Could you check a few things on this model? Use its own coordinates, in mm. A direction names the side the tool comes from. Coordinates: 2 decimals unless noted, no trailing zeros. Loops run counter-clockwise (first coordinate to the right, second up) from the corner with the lowest first, then second, coordinate; pieces in that order, holes last.
from build123d import *

# Parameters (mm, degrees)
SKETCH_R        = 40
SKETCH_R_2      = 1.7
PAD_DEPTH       = 5
POCKET_DEPTH    = 231.496033
CHAMFER_SIZE    = 2.5
SKETCH002_W     = 4
SKETCH002_H     = 20
PAD001_DEPTH    = 24
SKETCH003_R     = 2.2
POCKET001_DEPTH = 57.501
SKETCH004_R     = 1.75
POCKET002_DEPTH = 29.001
SKETCH005_R     = 2
POCKET003_DEPTH = 4
SKETCH006_R     = 2
POCKET004_DEPTH = 4
PAD002_DEPTH    = 2.5
SKETCH008_R     = 1.75
POCKET005_DEPTH = 262.590383
SKETCH009_R     = 2.85
POCKET006_DEPTH = 3
SKETCH015_W     = 4
SKETCH015_H     = 13
PAD003_DEPTH    = 12
POCKET007_DEPTH = 4
SKETCH017_W     = 2
SKETCH017_H     = 20
PAD004_DEPTH    = 40
SKETCH018_W     = 4
SKETCH018_H     = 10
PAD005_DEPTH    = 16
SKETCH019_W     = 16
SKETCH019_H     = 4
PAD006_DEPTH    = 4
SKETCH020_W     = 8.3
SKETCH020_H     = 3.5
SKETCH020_W_2   = 7.5
SKETCH020_H_2   = 4
POCKET008_DEPTH = 2
SKETCH021_W     = 4
SKETCH021_H     = 8
POCKET009_DEPTH = 15.001


with BuildPart() as part:
    # Sketch → Pad (new body)
    with BuildSketch(Plane.XY):
        Circle(SKETCH_R)
        with Locations((10, 10)):
            Circle(SKETCH_R_2, mode=Mode.SUBTRACT)
        with Locations((-10, 10)):
            Circle(SKETCH_R_2, mode=Mode.SUBTRACT)
        with Locations((-10, -10)):
            Circle(SKETCH_R_2, mode=Mode.SUBTRACT)
        with Locations((10, -10)):
            Circle(SKETCH_R_2, mode=Mode.SUBTRACT)
    extrude(amount=PAD_DEPTH)

    # Sketch001 → Pocket (cut, through all)
    with BuildSketch(Plane(origin=(0, 0, 0), x_dir=(1, 0, 0), z_dir=(0, 0, -1))):
        with BuildLine():
            ThreePointArc((22.5, 28.102491), (0, 36), (-22.5, 28.102491))
            Line((-22.5, 28.102491), (-12.5, 15.612495))
            ThreePointArc((12.5, 15.612495), (0, 20), (-12.5, 15.612495))
            Line((22.5, 28.102491), (12.5, 15.612495))
        make_face()
    pocket = extrude(amount=-POCKET_DEPTH, mode=Mode.SUBTRACT)

    # Mirrored: Pocket across Sketch001 H_Axis
    add(pocket.mirror(Plane(origin=(0, 0, 0), x_dir=(0, 0, -1), z_dir=(0, -1, 0))), mode=Mode.SUBTRACT)

    # Chamfer
    chamfer_edges = [part.edges().sort_by_distance(p)[0] for p in [
        (0, 20, 5),
        (17.5, 21.857493, 5),
        (0, 36, 5),
        (-17.5, 21.857493, 5),
        (-17.5, -21.857493, 5),
        (17.5, -21.857493, 5),
        (0, -20, 5),
        (0, -36, 5),
    ]]
    chamfer(chamfer_edges, length=CHAMFER_SIZE)

    # Sketch002 → Pad001 (new body)
    with BuildSketch(Plane.XY.offset(5)):
        with Locations((15.5, 0)):
            Rectangle(SKETCH002_W, SKETCH002_H)
        with Locations((-15.5, 0)):
            Rectangle(SKETCH002_W, SKETCH002_H)
    extrude(amount=PAD001_DEPTH)

    # Sketch003 → Pocket001 (cut, through all)
    with BuildSketch(Plane(origin=(-17.5, 0, 0), x_dir=(0, -1, 0), z_dir=(-1, 0, 0))):
        with Locations((0, 25)):
            Circle(SKETCH003_R)
    extrude(amount=-POCKET001_DEPTH, mode=Mode.SUBTRACT)

    # Sketch004 → Pocket002 (cut, through all)
    with BuildSketch(Plane(origin=(0, 0, 0), x_dir=(1, 0, 0), z_dir=(0, 0, -1))):
        with Locations((0, 13.5)):
            Circle(SKETCH004_R)
        with Locations((0, -13.5)):
            Circle(SKETCH004_R)
    extrude(amount=-POCKET002_DEPTH, mode=Mode.SUBTRACT)

    # Sketch005 → Pocket003 (cut)
    with BuildSketch(Plane.XY.offset(5)):
        with Locations((-10, 10)):
            Circle(SKETCH005_R)
        with Locations((10, 10)):
            Circle(SKETCH005_R)
        with Locations((10, -10)):
            Circle(SKETCH005_R)
        with Locations((-10, -10)):
            Circle(SKETCH005_R)
    extrude(amount=-POCKET003_DEPTH, mode=Mode.SUBTRACT)

    # Sketch006 → Pocket004 (cut)
    with BuildSketch(Plane(origin=(0, 0, 0), x_dir=(1, 0, 0), z_dir=(0, 0, -1))):
        with Locations((0, 13.5)):
            Circle(SKETCH006_R)
        with Locations((0, -13.5)):
            Circle(SKETCH006_R)
    extrude(amount=-POCKET004_DEPTH, mode=Mode.SUBTRACT)

    # Sketch007 → Pad002 (new body)
    with BuildSketch(Plane(origin=(0, 0, 0), x_dir=(1, 0, 0), z_dir=(0, 0, -1))):
        with BuildLine():
            ThreePointArc((16.875, 21.076868), (9.529651, 25.262339), (1.25, 26.971049))
            Line((1.25, 26.971049), (1.25, 19.960899))
            Line((-1.25, 19.960899), (1.25, 19.960899))
            Line((-1.25, 26.971049), (-1.25, 19.960899))
            ThreePointArc((-1.25, 26.971049), (-9.529651, 25.262339), (-16.875, 21.076868))
            Line((-18.4375, 23.02843), (-16.875, 21.076868))
            ThreePointArc((-1.25, 29.473505), (-10.357807, 27.621836), (-18.4375, 23.02843))
            Line((-1.25, 35.978292), (-1.25, 29.473505))
            ThreePointArc((1.25, 35.978292), (0, 36), (-1.25, 35.978292))
            Line((1.25, 35.978292), (1.25, 29.473505))
            ThreePointArc((18.4375, 23.02843), (10.357807, 27.621836), (1.25, 29.473505))
            Line((18.4375, 23.02843), (16.875, 21.076868))
        make_face()
    pad002 = extrude(amount=-PAD002_DEPTH)

    # Mirrored001: Pad002 across Sketch007 H_Axis
    add(pad002.mirror(Plane(origin=(0, 0, 0), x_dir=(0, 0, -1), z_dir=(0, -1, 0))))

    # Sketch008 → Pocket005 (cut, through all)
    with BuildSketch(Plane(origin=(0, 0, 0), x_dir=(1, 0, 0), z_dir=(0, 0, -1))):
        with Locations((26, 24)):
            Circle(SKETCH008_R)
        with Locations((26, -24)):
            Circle(SKETCH008_R)
    pocket005 = extrude(amount=-POCKET005_DEPTH, mode=Mode.SUBTRACT)

    # Mirrored002: Pocket005 across Sketch008 V_Axis
    add(pocket005.mirror(Plane(origin=(0, 0, 0), x_dir=(0, 0, -1), z_dir=(1, 0, 0))), mode=Mode.SUBTRACT)

    # Sketch009 → Pocket006 (cut)
    with BuildSketch(Plane(origin=(0, 0, 0), x_dir=(1, 0, 0), z_dir=(0, 0, -1))):
        with Locations((-26, 24)):
            Circle(SKETCH009_R)
        with Locations((-26, -24)):
            Circle(SKETCH009_R)
        with Locations((26, -24)):
            Circle(SKETCH009_R)
        with Locations((26, 24)):
            Circle(SKETCH009_R)
    extrude(amount=-POCKET006_DEPTH, mode=Mode.SUBTRACT)

    # Sketch015 → Pad003 (new body)
    with BuildSketch(Plane(origin=(-17.5, 0, 0), x_dir=(0, -1, 0), z_dir=(-1, 0, 0))):
        with Locations((0, 11.5)):
            Rectangle(SKETCH015_W, SKETCH015_H)
    extrude(amount=PAD003_DEPTH)

    # Sketch016 → Pocket007 (cut)
    with BuildSketch(Plane(origin=(0, 2, 0), x_dir=(-1, 0, 0), z_dir=(0, 1, 0))):
        Polygon((17.5, 18), (29.5, 18), (29.5, 5), align=None)
    extrude(amount=-POCKET007_DEPTH, mode=Mode.SUBTRACT)

    # Sketch017 → Pad004 (new body)
    with BuildSketch(Plane.XY.offset(5)):
        with Locations((34.5, 0)):
            Rectangle(SKETCH017_W, SKETCH017_H)
    extrude(amount=PAD004_DEPTH)

    # Sketch018 → Pad005 (new body)
    with BuildSketch(Plane.YZ.offset(17.5)):
        with Locations((0, 10)):
            Rectangle(SKETCH018_W, SKETCH018_H)
    extrude(amount=PAD005_DEPTH)

    # Sketch019 → Pad006 (new body)
    with BuildSketch(Plane.XY.offset(29)):
        with Locations((25.5, -8)):
            Rectangle(SKETCH019_W, SKETCH019_H)
        with Locations((25.5, 8)):
            Rectangle(SKETCH019_W, SKETCH019_H)
    extrude(amount=-PAD006_DEPTH)

    # Sketch020 → Pocket008 (cut)
    with BuildSketch(Plane.YZ.offset(35.5)):
        with Locations((0, 40.25)):
            Rectangle(SKETCH020_W, SKETCH020_H)
        with Locations((0, 26)):
            Rectangle(SKETCH020_W_2, SKETCH020_H_2)
    extrude(amount=-POCKET008_DEPTH, mode=Mode.SUBTRACT)

    # Sketch021 → Pocket009 (cut, through all)
    with BuildSketch(Plane.XY.offset(15)):
        with Locations((27, 0)):
            Rectangle(SKETCH021_W, SKETCH021_H)
    extrude(amount=-POCKET009_DEPTH, mode=Mode.SUBTRACT)


solid = part.part
1) For faces 1 (the flat face through (31, 0, 15)), 2 (the flat face through (35, 4.15, 40)), 3 (the flat face through (1.25, -24, 1)), 4 (the cylindrical face through (27.315, -21.472, 1.479)), 5 (the cylindrical face through (10, 12, 3)), which set-ups out of +Z, -Z, +X, -X, +Y, -Y let a thin tool reach every point of the face, with its end or its side?
2) We'd pull the mould along Y, two halves only. Please class faces 6 (the flat face through (-20.497, -25.601, 1.232)), 7 (the flat face through (21, 2, 10)), 8 (the flat face through (-1, 1, 5)): released by +Y, released by -Y, zero draft, split by the parting line, or undercut.
3) Will these pins go through, and if not, where does the flat tip stop? pin 1 (4.5 mm diameter, centred on x = -26, y = -24, fed in from +Z); pin 2 (1.7 mm diameter, centred on x = 26, y = 23, fed in from -Z); pin 3 (2 mm diameter, centred on x = -15, y = 1, fed in from +Z).
4) If I drill on L1, parallel to Y at x = 17, z = 23; L2, parallel to Z at x = -28, y = 20.5; L3, parallel to Y at x = 10, z = 4.15, over which ranges is the centre line in solid material (lowest first)?
5) Imagine slicing it at B-B on y = 0. State how many separate pieces and enclosed holes the cut face has, plus the area to 3 significant figures.
6) Imagine slicing it at A-A on z = 16. List the corners of the cut face in (x, y) for me, plus the area to 3 significant figures.
Solved:
1. face 1: +Z, +Y, -Y
1. face 2: +X, -X
1. face 3: +Z, -Z
1. face 4: -Z
1. face 5: +Z
2. face 6: undercut
2. face 7: released by +Y
2. face 8: zero draft
3. pin 1: stops at z = 5
3. pin 2: stops at z = 3
3. pin 3: stops at z = 29
4. L1: y = -10 to -0.92, 0.92 to 10
4. L2: z = 0 to 5
4. L3: y = -38.73 to -36.3, -15.39 to -12, -8 to 8, 12 to 15.39, 36.3 to 38.73
5. separate pieces: 6
5. enclosed holes: 0
5. area: 800 mm2
6. outline: (-19.35, -2) - (-17.5, -2) - (-17.5, -10) - (-13.5, -10) - (-13.5, 10) - (-17.5, 10) - (-17.5, 2) - (-19.35, 2) - close; (13.5, -10) - (17.5, -10) - (17.5, 10) - (13.5, 10) - close; (33.5, -10) - (35.5, -10) - (35.5, 10) - (33.5, 10) - close
6. area: 207 mm2
